```python
from build123d import *

# Parameters (mm, degrees)
ESQUISSE1_R              = 47.75
BOSS_EXTRU_1_DEPTH       = 50
ESQUISSE2_R              = 26
ENL_V_MAT_EXTRU_1_DEPTH  = 20
ESQUISSE3_R              = 11
ENL_V_MAT_EXTRU_5_DEPTH  = 7.5
ESQUISSE4_R              = 5
ENL_V_MAT_EXTRU_6_DEPTH  = 13.5
ESQUISSE11_R             = 2.75
ENL_V_MAT_EXTRU_11_DEPTH = 85.024549984
ESQUISSE12_R             = 47.75
ESQUISSE12_R_2           = 46.5
ENL_V_MAT_EXTRU_12_DEPTH = 85.024549984
ESQUISSE16_R             = 60
BOSS_EXTRU_3_DEPTH       = 50
ESQUISSE17_R             = 2.75
ENL_V_MAT_EXTRU_14_DEPTH = 128.377392029
ESQUISSE18_R             = 6
ENL_V_MAT_EXTRU_15_DEPTH = 4


with BuildPart() as part:
    # Esquisse1 → Boss.-Extru.1 (new body)
    with BuildSketch(Plane(origin=(0, 0, 0), x_dir=(1, 0, 0), z_dir=(0, 1, 0))):
        with Locations(Location((0, 0, 0), (0, 0, 270))):
            Circle(ESQUISSE1_R)
    extrude(amount=BOSS_EXTRU_1_DEPTH)

    # Esquisse2 → Enlèv. mat.-Extru.1 (cut)
    with BuildSketch(Plane(origin=(0, 0, 0), x_dir=(-1, 0, 0), z_dir=(0, -1, 0))):
        with Locations(Location((0, 0, 0), (0, 0, 90))):
            Circle(ESQUISSE2_R)
    extrude(amount=-ENL_V_MAT_EXTRU_1_DEPTH, mode=Mode.SUBTRACT)

    # Esquisse3 → Enlèv. mat.-Extru.5 (cut)
    with BuildSketch(Plane(origin=(0, 20, 0), x_dir=(-1, 0, 0), z_dir=(0, -1, 0))):
        with Locations(Location((0, 0, 0), (0, 0, 90))):
            Circle(ESQUISSE3_R)
    extrude(amount=-ENL_V_MAT_EXTRU_5_DEPTH, mode=Mode.SUBTRACT)

    # Esquisse4 → Enlèv. mat.-Extru.6 (cut)
    with BuildSketch(Plane(origin=(0, 27.5, 0), x_dir=(-1, 0, 0), z_dir=(0, -1, 0))):
        with Locations(Location((0, 0, 0), (0, 0, 90))):
            Circle(ESQUISSE4_R)
    extrude(amount=-ENL_V_MAT_EXTRU_6_DEPTH, mode=Mode.SUBTRACT)

    # Esquisse11 → Enlèv. mat.-Extru.11 (cut, through all)
    with BuildSketch(Plane(origin=(0, 50, 0), x_dir=(1, 0, 0), z_dir=(0, 1, 0))):
        with Locations(Location((-16, 0, 0), (0, 0, 270))):
            Circle(ESQUISSE11_R)
        with Locations(Location((0, 16, 0), (0, 0, 270))):
            Circle(ESQUISSE11_R)
        with Locations(Location((16, 0, 0), (0, 0, 270))):
            Circle(ESQUISSE11_R)
        with Locations(Location((0, -16, 0), (0, 0, 270))):
            Circle(ESQUISSE11_R)
    extrude(amount=-ENL_V_MAT_EXTRU_11_DEPTH, mode=Mode.SUBTRACT)

    # Esquisse12 → Enlèv. mat.-Extru.12 (cut, through all)
    with BuildSketch(Plane.XZ):
        Circle(ESQUISSE12_R)
        with Locations(Location((0, 0, 0), (0, 0, 270))):
            Circle(ESQUISSE12_R_2, mode=Mode.SUBTRACT)
    extrude(amount=-ENL_V_MAT_EXTRU_12_DEPTH, mode=Mode.SUBTRACT)

    # Enlèv. mat.-Surface1
    split(bisect_by=Plane(origin=(0, 45, 0), x_dir=(1, 0, 0), z_dir=(0, 1, 0)), keep=Keep.BOTTOM)

    # Esquisse16 → Boss.-Extru.3 (add)
    with BuildSketch(Plane(origin=(0, 45, 0), x_dir=(1, 0, 0), z_dir=(0, 1, 0))):
        with Locations(Location((0, 0, 0), (0, 0, 270))):
            Circle(ESQUISSE16_R)
    extrude(amount=BOSS_EXTRU_3_DEPTH)

    # Esquisse17 → Enlèv. mat.-Extru.14 (cut, through all)
    with BuildSketch(Plane(origin=(0, 95, 0), x_dir=(1, 0, 0), z_dir=(0, 1, 0))):
        with Locations(Location((0, -16, 0), (0, 0, 270))):
            Circle(ESQUISSE17_R)
        with Locations(Location((-16, 0, 0), (0, 0, 270))):
            Circle(ESQUISSE17_R)
        with Locations(Location((0, 16, 0), (0, 0, 270))):
            Circle(ESQUISSE17_R)
        with Locations(Location((16, 0, 0), (0, 0, 270))):
            Circle(ESQUISSE17_R)
    extrude(amount=-ENL_V_MAT_EXTRU_14_DEPTH, mode=Mode.SUBTRACT)

    # Esquisse18 → Enlèv. mat.-Extru.15 (cut)
    with BuildSketch(Plane(origin=(0, 95, 0), x_dir=(1, 0, 0), z_dir=(0, 1, 0))):
        with Locations(Location((0, 16, 0), (0, 0, 270))):
            Circle(ESQUISSE18_R)
        with Locations(Location((16, 0, 0), (0, 0, 270))):
            Circle(ESQUISSE18_R)
        with Locations(Location((0, -16, 0), (0, 0, 270))):
            Circle(ESQUISSE18_R)
        with Locations(Location((-16, 0, 0), (0, 0, 270))):
            Circle(ESQUISSE18_R)
    extrude(amount=-ENL_V_MAT_EXTRU_15_DEPTH, mode=Mode.SUBTRACT)


solid = part.part
```
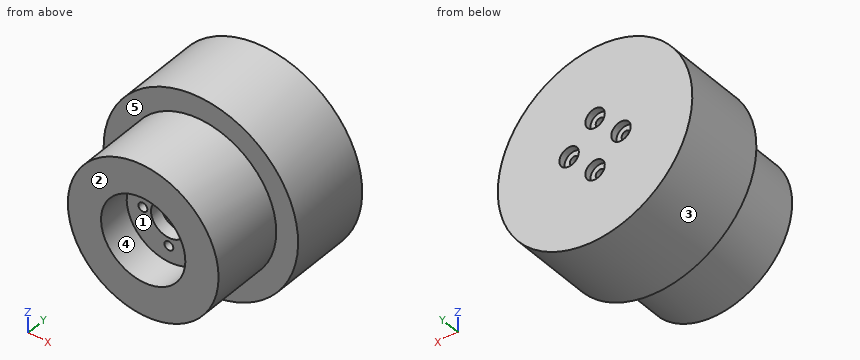
The model under review builds one solid part; all positions refer to its coordinate system, in mm. Face numbers are marked on the shaded views. A direction names the side the tool comes from. Round coordinates to 2 decimals unless told otherwise and drop trailing zeros. Write each loop counter-clockwise with the first axis right and the second up, starting at its lowest first coordinate (ties: lowest second). Pieces come first, ordered by that corner, then holes. Notation, with made-up numbers: (88, -13.5) - (144, -13.5) arc R8 cw to (144, -0.5) - close; hole circle Ø9 at (18.5, 17.5). An arc over 180 degrees is marked (long way). Answer as CSV lines item,"result". Start each with the question number.
(1) We need section C-C on z = 0. Give the number of separate pieces and of enclosed holes in the cut face, plus the area to 3 significant figures.
(2) To check wall thickness, follow line 1 (X direction, y = 32, z = 0); line 2 (Y direction, x = 8.5, z = -14); line 3 (Y direction, x = -45.5, z = -20.5). State the ranges of each line that lie inside material, in increasing order.
(3) We need section B-B on x = -16. State the section outline as (y, z) points, plus the area to 3 significant figures.
(4) We need section D-D on z = 16. State the section outline as (x, y) points, plus the area to 3 significant figures.
(5) For pin 1 Ø12 at (y, z) = (36, -37) entering from -X; pin 2 Ø1.5 at (y, z) = (79.5, -29.5) entering from +X; pin 3 Ø2 at (x, y) = (-15.5, 15.5) entering from -Z, all flat-tipped, find the tip position at first contact; note any pin that passes through.
(6) Draft analysis for pull direction X (two halves, no side actions). For the marked faces 3, 4 and 5, state which applies: pulls with the +X half, pulls with the -X half, needs draft (parallel to the pull), parting line crosses it, or undercut.
(7) For the marked faces 1 and 2, list the 3-axis set-ups (+Z, -Z, +X, -X, +Y, -Y) from which the entire face can be reached by the end or side of a thin tool; tool diameter is ignored.
(8) We need section A-A on y = 36. State the section outline as (x, z) points.
Worked answers:
1,separate pieces,"3"
1,enclosed holes,"0"
1,area,"7,970 mm²"
2,line 1,"-46.5 to -18.75, -13.25 to -5, 5 to 13.25, 18.75 to 46.5"
2,line 2,"20 to 95"
2,line 3,"45 to 95"
3,outline,"(0, -43.66) - (45, -43.66) - (45, -57.83) - (95, -57.83) - (95, -6) - (91, -6) - (91, -2.75) - (20, -2.75) - (20, -20.49) - (0, -20.49) - close; (0, 20.49) - (20, 20.49) - (20, 2.75) - (91, 2.75) - (91, 6) - (95, 6) - (95, 57.83) - (45, 57.83) - (45, 43.66) - (0, 43.66) - close"
3,area,"8,450 mm²"
4,outline,"(-57.83, 45) - (-43.66, 45) - (-43.66, 0) - (-20.49, 0) - (-20.49, 20) - (-2.75, 20) - (-2.75, 91) - (-6, 91) - (-6, 95) - (-57.83, 95) - close; (2.75, 20) - (20.49, 20) - (20.49, 0) - (43.66, 0) - (43.66, 45) - (57.83, 45) - (57.83, 95) - (6, 95) - (6, 91) - (2.75, 91) - close"
4,area,"8,450 mm²"
5,pin 1,"x = -34.66"
5,pin 2,"x = 52.66"
5,pin 3,"z = -44.18"
6,face 3,"parting line crosses it"
6,face 4,"undercut"
6,face 5,"needs draft"
7,face 1,"-Y"
7,face 2,"+Z, -Z, +X, -X, -Y"
8,outline,"circle Ø93 at (0, 0); hole circle Ø5.5 at (-16, 0); hole circle Ø10 at (0, 0); hole circle Ø5.5 at (0, -16); hole circle Ø5.5 at (0, 16); hole circle Ø5.5 at (16, 0)"
